CAD build for the part. Positions are in the model's coordinates, mm. Face numbers are marked on the shaded views. A direction names the side the tool comes from. Round coordinates to 2 decimals unless told otherwise and drop trailing zeros. Loops run counter-clockwise (first coordinate to the right, second up) from the corner with the lowest first, then second, coordinate; pieces in that order, holes last. Notation, with made-up numbers: M 61.5,32 L 114.5,32 A27 ccw 114.5,56 Z; hole C 25.5,-25 d6. An arc over 180 degrees is marked long. Use one line per item in the form item = value.
from build123d import *

# Parameters (mm, degrees)
F1_DEPTH = 14
F2_R     = 1.75
F3_DEPTH = 2.501
F4_R     = 1.75
F5_DEPTH = 25
F6_R     = 3


with BuildPart() as f1:
    # F0 (on Front) → F1 (new body)
    with BuildSketch(Plane.XZ):
        Polygon((-14, 0), (0, 0), (0, 21), (21, 21), (21, 35), (18.5, 35), (18.5, 23.5), (-2.5, 23.5), (-2.5, 2.5), (-14, 2.5), align=None)
    extrude(amount=F1_DEPTH)

    # F2 (on face) → F3 (cut, through all)
    with BuildSketch(Plane(origin=(18.5, 0, 0), x_dir=(0, -1, 0), z_dir=(-1, 0, 0))):
        with Locations((7, 29.25)):
            Circle(F2_R)
    extrude(amount=-F3_DEPTH, mode=Mode.SUBTRACT)

    # F4 (on face) → F5 (cut)
    with BuildSketch(Plane.XY.offset(2.5)):
        with Locations((-8.25, -7)):
            Circle(F4_R)
    extrude(amount=-F5_DEPTH, mode=Mode.SUBTRACT)

    # F6
    f6_edges = [f1.edges().sort_by_distance(p)[0] for p in [
        (-14, -14, 1.25),
        (-14, 0, 1.25),
        (19.75, -14, 35),
        (19.75, 0, 35),
    ]]
    fillet(f6_edges, radius=F6_R)


solid = f1.part
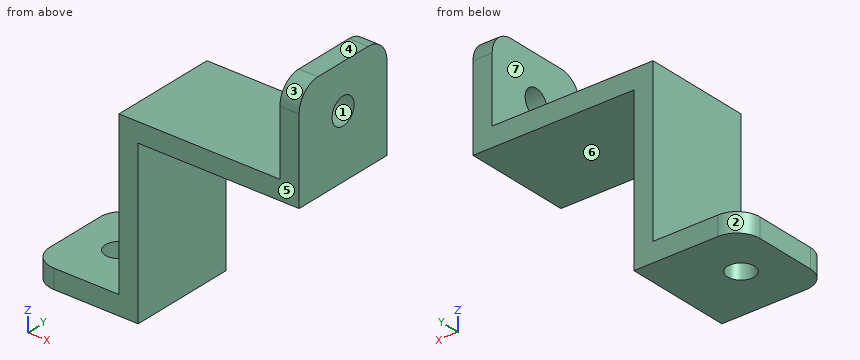
1. Cut at D-D on y = -4.5. Write the cut outline in (x, z).
Completed:
outline = M -14,0 L 0,0 L 0,21 L 21,21 L 21,35 L 18.5,35 L 18.5,23.5 L -2.5,23.5 L -2.5,2.5 L -14,2.5 Z
2. Cut at C-C on x = -8.25. Write the cut outline in (y, z), and give its area (4 significant figures).
Completed:
outline = M -14,0 L -8.75,0 L -8.75,2.5 L -14,2.5 Z; M -5.25,0 L 0,0 L 0,2.5 L -5.25,2.5 Z
area = 26.25 mm2
3. Tool access for the marked faces 5, 6 and 7: list every direction of +Z, -Z, +X, -X, +Y, -Y with a clear straight run to the whole face (end or side of a thin tool).
Completed:
face_5 = +Z, -Z, +X, -X, -Y
face_6 = -Z, +X, +Y, -Y
face_7 = +Z, -X, +Y, -Y
4. Pull direction Y, two halves, no side cores. Call the marked faces 1, 2, 3 and 4: +Y half, -Y half, draft (parallel to the pull), parting line (faces both ways), or undercut.
Completed:
face_1 = undercut
face_2 = +Y half
face_3 = -Y half
face_4 = draft
5. Cut at B-B on y = -7. Write the cut outline in (x, z), and give its area (3 significant figures).
Completed:
outline = M -14,0 L -10,0 L -10,2.5 L -14,2.5 Z; M -6.5,0 L 0,0 L 0,21 L 21,21 L 21,27.5 L 18.5,27.5 L 18.5,23.5 L -2.5,23.5 L -2.5,2.5 L -6.5,2.5 Z; M 18.5,31 L 21,31 L 21,35 L 18.5,35 Z
area = 151 mm2
6. Drop flat-ended pins along their axis: P1, Ø3.5, axis at x = -7.5, y = -8.5, coming from the +Z side; P2, Ø1.5, axis at y = -4.5, z = 11.5, coming from the +X side; P3, Ø3, axis at y = -7, z = 29.25, coming from the -X side; P4, Ø7, axis at x = 14.5, y = -9, coming from the -Z side. Give the stop position or say it passes through.
Completed:
P1 = 2.5
P2 = 0
P3 = through
P4 = 21
7. Probe line 1 along Z through (x, y) = (19.25, -7); line 2 along Y through (x, z) = (-8.25, 0.75); line 3 along X through (y, z) = (-1.75, 15). List the from-to ranges inside material, lowest first. Write a range as from..to.
Completed:
line_1 = 21..27.5, 31..35
line_2 = -14..-8.75, -5.25..0
line_3 = -2.5..0
8. Cut at A-A on z = 29.25. Write the cut outline in (x, y).
Completed:
outline = M 18.5,-14 L 21,-14 L 21,-8.75 L 18.5,-8.75 Z; M 18.5,-5.25 L 21,-5.25 L 21,0 L 18.5,0 Z
